Geometry: final body of the model. Coordinates: model frame, mm. A direction names the side the tool comes from. Give positions to 0.01 mm unless a question says otherwise; leave off trailing zeros. Write each loop counter-clockwise with the first axis right and the second up, starting at its lowest first coordinate (ties: lowest second). Pieces come first, ordered by that corner, then holes. Notation, with made-up numbers: M 46,-8.5 L 66,-8.5 A25 ccw 66,14.5 Z; hole C 71.25,-25.75 d3. An arc over 180 degrees is marked long. Use a Markdown table: item, result. Add a question column.
1) Draft query along X for faces 1 (the flat face through (0, 40, 0)), 2 (the flat face through (-23.5, 16, 35)), 3 (the cylindrical face through (34.9, 10.57, 35.46)), 4 (the flat face through (32.5, 37, 35)). Return one class per face: +X half, -X half, draft (parallel to the pull), parting line (faces both ways), or undercut.
2) Section C-C on x = 9. Return the cut outline in (y, z).
3) Section A-A on y = 33. Return the cut outline in (x, z), then the cut area to 3 significant figures.
4) Pin query (flat end, axial travel): pin 1 (10 mm diameter, centred on x = 1.5, z = 59, fed in from +Y); pin 2 (2 mm diameter, centred on x = 20, z = 39, fed in from -Y); pin 3 (11 mm diameter, centred on x = 1.5, z = 24.5, fed in from -Y). Return the tip coordinate at first contact, or that it passes through.
5) Set-up query: faces 5 (the cylindrical face through (31.9, 37.82, 3.57)), 6 (the cylindrical face through (-19.9, 19.43, 35.46)), 7 (the cylindrical face through (21.07, 15.04, 0.6)). Return all of +Z, -Z, +X, -X, +Y, -Y with unobstructed straight access to the full face (end or side cutting, diameter ignored); none if empty.
6) Line query: line 1 (X direction, y = 15, z = 17.5); line 2 (X direction, y = 57, z = 52); line 3 (Z direction, x = -28.5, y = 16.5). Output: solid intervals per line, ascending.
```python
from build123d import *

# Parameters (mm, degrees)
BOSS_EXTRU_2_DEPTH = 70
CONG_4_R           = 2
CONG_3_R           = 2
CONG_5_R           = 2
CONG_6_R           = 2
COQUE1_START       = 3
COQUE1_DEPTH       = 64
CONG_7_R           = 2
CONG_8_R           = 2
CONG_11_R          = 2
CONG_12_R          = 2
CONG_13_R          = 2


# Read off the part's stored shape, not the designer's step: Coque1
with BuildPart() as part:
    # Esquisse2 → Boss.-Extru.2 (new body)
    with BuildSketch(Plane.XY):
        Polygon((-35.5, 10), (-20.5, 10), (-20.5, 20), (20.5, 20), (20.5, 10), (35.5, 10), (35.5, 60), (-35.5, 60), align=None)
    extrude(amount=BOSS_EXTRU_2_DEPTH)

    # Congé4
    cong_4_edges = [part.edges().sort_by_distance(p)[0] for p in [
        (-35.5, 60, 35),
    ]]
    fillet(cong_4_edges, radius=CONG_4_R)

    # Congé3
    cong_3_edges = [part.edges().sort_by_distance(p)[0] for p in [
        (35.5, 60, 35),
    ]]
    fillet(cong_3_edges, radius=CONG_3_R)

    # Congé5
    cong_5_edges = [part.edges().sort_by_distance(p)[0] for p in [
        (20.5, 20, 35),
    ]]
    fillet(cong_5_edges, radius=CONG_5_R)

    # Congé6
    cong_6_edges = [part.edges().sort_by_distance(p)[0] for p in [
        (-20.5, 20, 35),
    ]]
    fillet(cong_6_edges, radius=CONG_6_R)

    # Coque1 outline → Coque1 (cut)
    with BuildSketch(Plane.XY.offset(COQUE1_START)):
        with BuildLine():
            Line((-32.5, 60), (-32.5, 13))
            Line((-32.5, 13), (-23.5, 13))
            Line((-23.5, 13), (-23.5, 18))
            ThreePointArc((-23.5, 18), (-22.035533906, 21.535533906), (-18.5, 23))
            Line((-18.5, 23), (18.5, 23))
            ThreePointArc((18.5, 23), (22.035533906, 21.535533906), (23.5, 18))
            Line((23.5, 18), (23.5, 13))
            Line((23.5, 13), (32.5, 13))
            Line((32.5, 13), (32.5, 60))
            Line((32.5, 60), (-32.5, 60))
        make_face()
    extrude(amount=COQUE1_DEPTH, mode=Mode.SUBTRACT)

    # Congé7
    cong_7_edges = [part.edges().sort_by_distance(p)[0] for p in [
        (35.5, 34, 0),
        (34.914213562, 59.414213562, 0),
        (0, 60, 0),
        (-34.914213562, 59.414213562, 0),
        (-28, 10, 0),
        (-35.5, 10, 35),
        (-35.5, 34, 0),
    ]]
    fillet(cong_7_edges, radius=CONG_7_R)

    # Congé8
    cong_8_edges = [part.edges().sort_by_distance(p)[0] for p in [
        (-20.5, 14, 70),
        (35.5, 10, 36),
        (20.5, 10, 35),
        (-20.5, 10, 36),
        (28, 10, 70),
        (35.5, 34, 70),
        (-35.5, 35, 70),
        (-34.914213562, 59.414213562, 70),
        (0, 60, 70),
        (34.914213562, 59.414213562, 70),
        (20.5, 14, 0),
        (20.5, 14, 70),
        (19.914213562, 19.414213562, 0),
        (19.914213562, 19.414213562, 70),
        (0, 20, 0),
        (0, 20, 70),
        (-19.914213562, 19.414213562, 0),
        (-19.914213562, 19.414213562, 70),
        (-20.5, 15, 0),
        (34.914213562, 10, 0.585786438),
        (-27, 10, 70),
        (-20.5, 10.585786438, 0.585786438),
        (-34.914213562, 10.585786438, 70),
        (27, 10, 0),
    ]]
    fillet(cong_8_edges, radius=CONG_8_R)

    # Congé11
    cong_11_edges = [part.edges().sort_by_distance(p)[0] for p in [
        (-23.5, 15.5, 3),
        (0, 23, 3),
        (23.5, 15.5, 3),
        (-23.5, 15.5, 67),
        (-22.035533906, 21.535533906, 67),
        (0, 23, 67),
        (22.035533906, 21.535533906, 67),
        (23.5, 15.5, 67),
        (22.035533906, 21.535533906, 3),
        (-22.035533906, 21.535533906, 3),
    ]]
    fillet(cong_11_edges, radius=CONG_11_R)

    # Congé12
    cong_12_edges = [part.edges().sort_by_distance(p)[0] for p in [
        (-32.5, 36.5, 3),
        (32.5, 36.5, 3),
        (32.5, 36.5, 67),
        (-32.5, 36.5, 67),
    ]]
    fillet(cong_12_edges, radius=CONG_12_R)

    # Congé13
    cong_13_edges = [part.edges().sort_by_distance(p)[0] for p in [
        (-23.5, 13, 35),
        (28, 13, 67),
        (-24.085786438, 13, 3.585786438),
        (-24.085786438, 13, 66.414213562),
        (23.5, 13, 35),
        (28, 13, 3),
        (24.085786438, 13, 3.585786438),
        (24.085786438, 13, 66.414213562),
        (-32.5, 13, 35),
        (-28, 13, 67),
        (-28, 13, 3),
        (-31.914213562, 13, 3.585786438),
        (-31.914213562, 13, 66.414213562),
        (32.5, 13, 35),
        (31.914213562, 13, 3.585786438),
        (31.914213562, 13, 66.414213562),
    ]]
    fillet(cong_13_edges, radius=CONG_13_R)


solid = part.part
```
Found:
| question | item | result |
|---|---|---|
| 1 | face 1 | draft |
| 1 | face 2 | undercut |
| 1 | face 3 | +X half |
| 1 | face 4 | undercut |
| 2 | outline | M 20,2 A2 ccw 22,0 L 58,0 A2 ccw 60,2 L 60,3 L 25,3 A2 cw 23,5 L 23,65 A2 cw 25,67 L 60,67 L 60,68 A2 ccw 58,70 L 22,70 A2 ccw 20,68 Z |
| 3 | outline | M -35.5,2 A2 ccw -33.5,0 L 33.5,0 A2 ccw 35.5,2 L 35.5,68 A2 ccw 33.5,70 L -33.5,70 A2 ccw -35.5,68 Z; hole M -32.5,5 A2 ccw -30.5,3 L 30.5,3 A2 ccw 32.5,5 L 32.5,65 A2 ccw 30.5,67 L -30.5,67 A2 ccw -32.5,65 Z |
| 3 | area | 810 mm² |
| 4 | pin 1 | y = 23 |
| 4 | pin 2 | y = 10.68 |
| 4 | pin 3 | y = 20 |
| 5 | face 5 | +Y |
| 5 | face 6 | +Z, -Z, -Y |
| 5 | face 7 | -Z, -Y |
| 6 | line 1 | -35.5 to -32.5, -23.5 to -20.5, 20.5 to 23.5, 32.5 to 35.5 |
| 6 | line 2 | -35.5 to -32.5, 32.5 to 35.5 |
| 6 | line 3 | 0 to 3, 67 to 70 |
